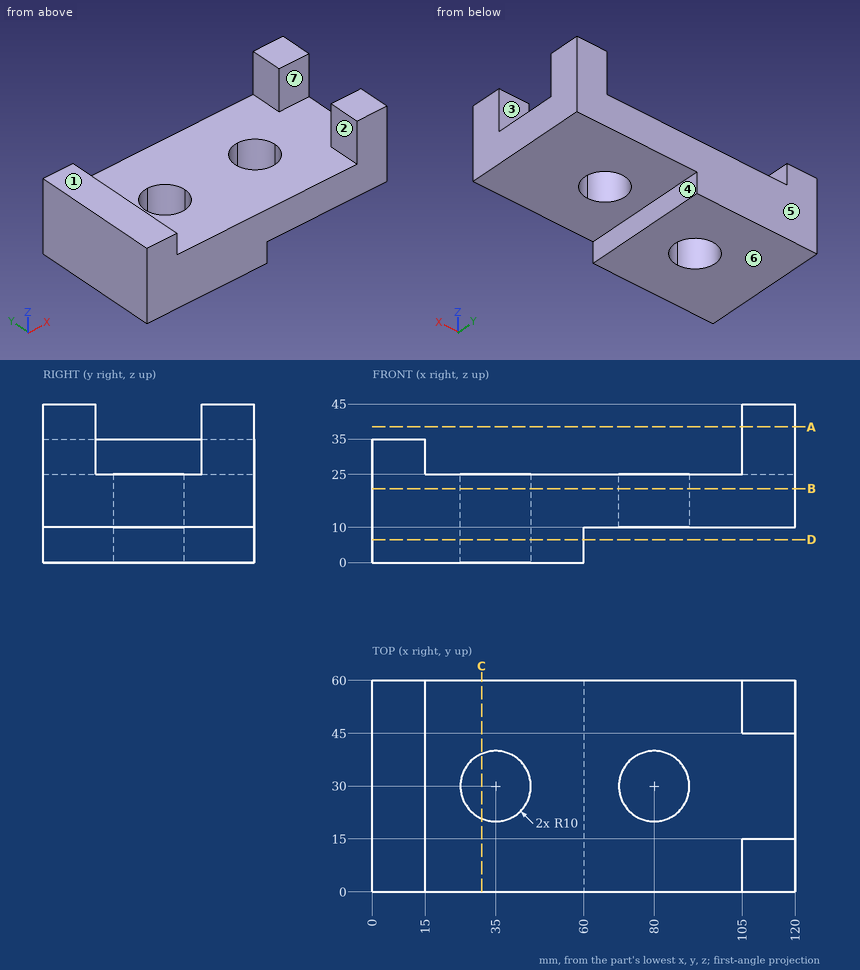
Geometry: see drawing. Coordinates: mm, zero at the bounding-box minimum. A direction names the side the tool comes from. Round coordinates to 2 decimals unless told otherwise and drop trailing zeros. Loops run counter-clockwise (first coordinate to the right, second up) from the corner with the lowest first, then second, coordinate; pieces in that order, holes last. Notation, with made-up numbers: M -13,79 L -8,79 A17 ccw -8,87 Z; hole C 39.25,29 d3. An arc over 180 degrees is marked long. Use a Markdown table: item, result. Add a question column.
1. Ray query, line 1 along X through (y, z) = (34, 19); line 2 along X through (y, z) = (33, 14); line 3 along X through (y, z) = (46.5, 27). Return the intervals inside material, ascending. Write a range as [from, to].
2. Contact query for flat-ended pins moving along their axis: pin 1 (5 mm diameter, centred on x = 84, y = 19.5, fed in from +Z); pin 2 (16.5 mm diameter, centred on x = 4.5, y = 31.5, fed in from +Z); pin 3 (1.5 mm diameter, centred on x = 85, y = 21, fed in from -Z); pin 4 (6 mm diameter, centred on x = 24.5, y = 12.5, fed in from -Z). Output: stop coordinate, or through.
3. Cut plane C-C, the plane x = 31. Output: boundary loops of the cut face in (y, z), and give its area (3 significant figures).
4. Cut plane D-D, the plane z = 6.5. Output: boundary loops of the cut face in (x, y), and give its area (3 significant figures).
5. Cut plane A-A, the plane z = 38.5. Output: boundary loops of the cut face in (x, y), and give its area (3 significant figures).
6. Pull-direction query (Y, two-part tool) for the marked faces 5, 6 and 7; classes: +Y half, -Y half, draft (parallel to the pull), parting line (faces both ways), or undercut.
7. Cut plane B-B, the plane z = 21. Output: boundary loops of the cut face in (x, y).
8. Set-up query: the marked faces 1, 2, 3 and 4. Return all of +Z, -Z, +X, -X, +Y, -Y with unobstructed straight access to the full face (end or side cutting, diameter ignored); none if empty.
Solution:
| question | item | result |
|---|---|---|
| 1 | line 1 | x = [0, 25.83], [44.17, 70.83], [89.17, 120] |
| 1 | line 2 | x = [0, 25.46], [44.54, 70.46], [89.54, 120] |
| 1 | line 3 | x = [0, 15], [105, 120] |
| 2 | pin 1 | stops at z = 25 |
| 2 | pin 2 | stops at z = 35 |
| 2 | pin 3 | stops at z = 10 |
| 2 | pin 4 | stops at z = 0 |
| 3 | outline | M 0,0 L 20.83,0 L 20.83,25 L 0,25 Z; M 39.17,0 L 60,0 L 60,25 L 39.17,25 Z |
| 3 | area | 1,040 mm2 |
| 4 | outline | M 0,0 L 60,0 L 60,60 L 0,60 Z; hole C 35,30 d20 |
| 4 | area | 3,290 mm2 |
| 5 | outline | M 105,0 L 120,0 L 120,15 L 105,15 Z; M 105,45 L 120,45 L 120,60 L 105,60 Z |
| 5 | area | 450 mm2 |
| 6 | face 5 | +Y half |
| 6 | face 6 | draft |
| 6 | face 7 | undercut |
| 7 | outline | M 0,0 L 120,0 L 120,60 L 0,60 Z; hole C 35,30 d20; hole C 80,30 d20 |
| 8 | face 1 | +Z, -X, +Y, -Y |
| 8 | face 2 | +Z, +Y, -Y |
| 8 | face 3 | +Z, +X |
| 8 | face 4 | -Z, +X, +Y, -Y |
